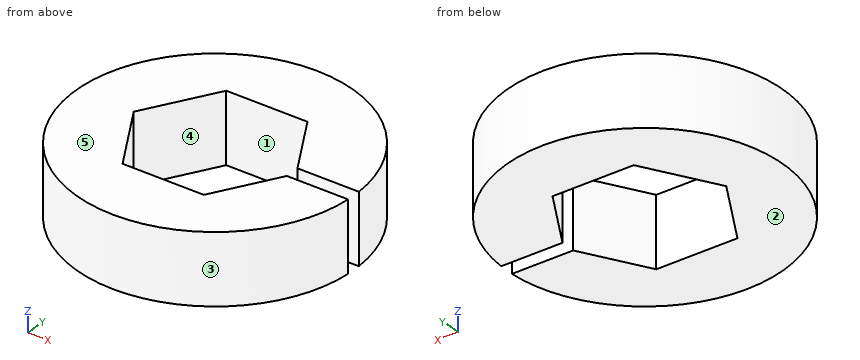
from build123d import *

# Parameters (mm, degrees)
SKETCH1_R           = 12.5
BOSS_EXTRUDE1_DEPTH = 6.33
SKETCH2_W           = 8.461167653
SKETCH2_H           = 1.32394958
CUT_EXTRUDE1_DEPTH  = 7.33


with BuildPart() as part:
    # Sketch1 → Boss-Extrude1 (new body)
    with BuildSketch(Plane.XY):
        Circle(SKETCH1_R)
        Polygon((7.332348419, 0), (3.666174209, 6.35), (-3.666174209, 6.35), (-7.332348419, 0), (-3.666174209, -6.35), (3.666174209, -6.35), align=None, mode=Mode.SUBTRACT)
    extrude(amount=BOSS_EXTRUDE1_DEPTH)

    # Sketch2 → Cut-Extrude1 (cut, through all)
    with BuildSketch(Plane.XY.offset(6.33)):
        with Locations((10.426813654, 0.014294586)):
            Rectangle(SKETCH2_W, SKETCH2_H)
    extrude(amount=-CUT_EXTRUDE1_DEPTH, mode=Mode.SUBTRACT)


solid = part.part
Input: part model. Units: mm. Frame: model coordinates. Face numbers are marked on the shaded views. A direction names the side the tool comes from. Round coordinates to 2 decimals unless told otherwise and drop trailing zeros. Loops run counter-clockwise (first coordinate to the right, second up) from the corner with the lowest first, then second, coordinate; pieces in that order, holes last. Notation, with made-up numbers: (11, 17) -> (46, 17) arc R20 ccw to (46, 22) -> close; hole circle Ø10 at (64, 25). An arc over 180 degrees is marked (long way). Answer as a JSON object with one key per item and string values. Group by question number.
1) Section query C-C on y = 2.75. Output: boundary loops of the cut face in (x, z), plus the area to 3 significant figures.
2) Section query A-A on x = 0. Output: boundary loops of the cut face in (y, z), plus the area to 3 significant figures.
3) Section query B-B on z = 6. Output: boundary loops of the cut face in (x, y), plus the area to 3 significant figures.
4) Draft query along X for the marked faces 3, 4 and 5. Return one class per face: +X half, -X half, draft (parallel to the pull), parting line (faces both ways), or undercut.
5) Reachability of the marked faces 1 and 2 from +Z, -Z, +X, -X, +Y, -Y: full face, straight path, thin tool, end or side. Return the list, or none.
6) Ray query, L1, parallel to X at y = -6.25, z = 4.5; L2, parallel to X at y = -4.5, z = 4; L3, parallel to Y at x = 10.75, z = 3.75. Return the intervals inside material, ascending.
7) Pin query (flat end, axial travel): pin 1 (2 mm diameter, centred on x = -7, z = 5.5, fed in from +Y); pin 2 (3 mm diameter, centred on x = -2.5, z = 4, fed in from +Y); pin 3 (1.5 mm diameter, centred on y = -1.5, z = 3, fed in from +X); pin 4 (1.5 mm diameter, centred on x = -3, y = -6, fed in from -Z). Return the tip coordinate at first contact, or that it passes through.
8) Section query D-D on y = 7.5. Output: boundary loops of the cut face in (x, z).
Reply:
{
 "1": {"outline": "(-12.19, 0) -> (-5.74, 0) -> (-5.74, 6.33) -> (-12.19, 6.33) -> close; (5.74, 0) -> (12.19, 0) -> (12.19, 6.33) -> (5.74, 6.33) -> close", "area": "81.6 mm2"},
 "2": {"outline": "(-12.5, 0) -> (-6.35, 0) -> (-6.35, 6.33) -> (-12.5, 6.33) -> close; (6.35, 0) -> (12.5, 0) -> (12.5, 6.33) -> (6.35, 6.33) -> close", "area": "77.9 mm2"},
 "3": {"outline": "(-7.33, 0) -> (-3.67, 6.35) -> (3.67, 6.35) -> (6.94, 0.68) -> (12.48, 0.68) arc R12.5 ccw (long way) to (12.48, -0.65) -> (6.96, -0.65) -> (3.67, -6.35) -> (-3.67, -6.35) -> close", "area": "344 mm2"},
 "4": {"face 3": "parting line", "face 4": "undercut", "face 5": "draft"},
 "5": {"face 1": "+Z, -Z", "face 2": "-Z, +X, -X, +Y, -Y"},
 "6": {"L1": "x = -10.83 to -3.72, 3.72 to 10.83", "L2": "x = -11.66 to -4.73, 4.73 to 11.66", "L3": "y = -6.38 to -0.65, 0.68 to 6.38"},
 "7": {"pin 1": "stops at y = 10.97", "pin 2": "stops at y = 12.46", "pin 3": "stops at x = 12.48", "pin 4": "stops at z = 0"},
 "8": {"outline": "(-10, 0) -> (10, 0) -> (10, 6.33) -> (-10, 6.33) -> close"}
}
